Here's the drawing with two shaded views (mm, measured from the low corner). I have some questions. Coordinates: 2 decimals unless noted, no trailing zeros. Loops run counter-clockwise (first coordinate to the right, second up) from the corner with the lowest first, then second, coordinate; pieces in that order, holes last. Notation, with made-up numbers: (64, 76.25) -> (88, 76.25) arc R8 cw to (88, 90.25) -> close; hole circle Ø11 at (-16.5, 64). An arc over 180 degrees is marked (long way). Answer as a JSON object with one key per item and string values. Group by question number.
Q1. I want a section at A-A on x = 136. Write out the boundary of the cut face in (y, z).
Q2. I want a section at B-B on z = 12.75. Write out the boundary of the cut face in (x, y).
Q3. I need wall thicknesses on line 1 (X direction, y = 3.25, z = 5.5); line 2 (Y direction, x = 136.5, z = 15.5); line 3 (Z direction, x = 108.5, y = 1). Which ranges of each line are inside material? Lowest first, please.
Q4. I'm going to push flat-ended pins straight in: pin 1 (8.5 mm diameter, centred on x = 52, z = 7, fed in from -Y); pin 2 (2 mm diameter, centred on x = 80.5, y = 1, fed in from +Z); pin 3 (0.8 mm diameter, centred on x = 80.5, y = 4, fed in from +Z); pin 4 (1.6 mm diameter, centred on y = 0.5, z = 9, fed in from +X). Where does each tip first touch, or does it pass through?
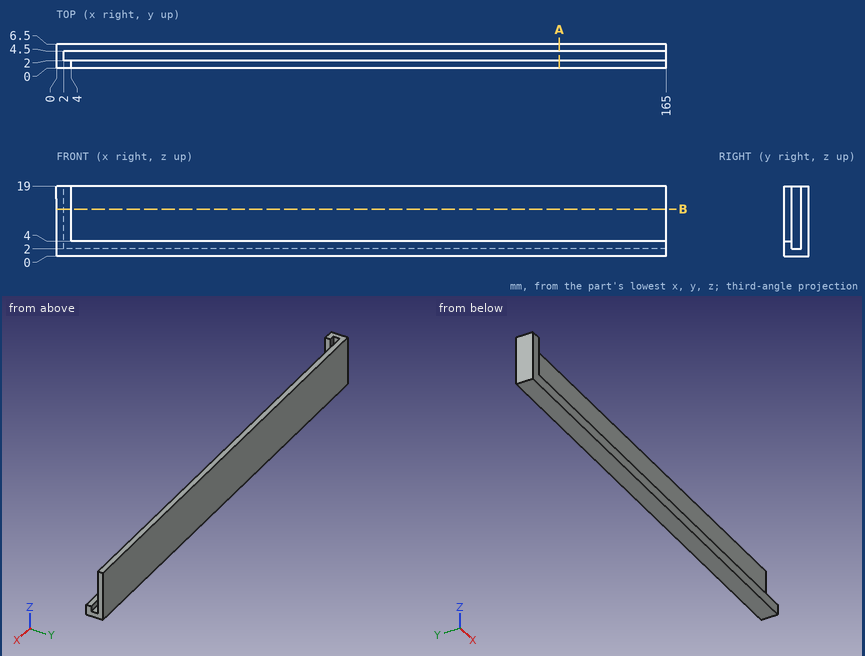
Result set:
{
 "1": {"outline": "(0, 0) -> (6.5, 0) -> (6.5, 19) -> (4.5, 19) -> (4.5, 2) -> (2, 2) -> (2, 4) -> (0, 4) -> close"},
 "2": {"outline": "(0, 0) -> (4, 0) -> (4, 2) -> (2, 2) -> (2, 4.5) -> (165, 4.5) -> (165, 6.5) -> (0, 6.5) -> close"},
 "3": {"line 1": "x = 0 to 2", "line 2": "y = 4.5 to 6.5", "line 3": "z = 0 to 4"},
 "4": {"pin 1": "stops at y = 0", "pin 2": "stops at z = 4", "pin 3": "stops at z = 2", "pin 4": "stops at x = 4"}
}
